```python
from build123d import *

# Parameters (mm, degrees)
SKETCH1_W                      = 3
SKETCH1_H                      = 76
BOSS_EXTRUDE1_DEPTH            = 220
M3_CLEARANCE_HOLE1_D           = 3.4
M3_CLEARANCE_HOLE1_CSINK_D     = 3.45
M3_CLEARANCE_HOLE1_CSINK_ANGLE = 90
SKETCH4_W                      = 220
SKETCH4_H                      = 15
CUT_EXTRUDE1_DEPTH             = 233.776717049
SKETCH5_R                      = 1.75
CUT_EXTRUDE2_DEPTH             = 233.776717049
BOSS_EXTRUDE2_START            = -3
SKETCH6_R                      = 1.725
SKETCH6_R_2                    = 1.7
BOSS_EXTRUDE2_DEPTH            = 3
BOSS_EXTRUDE3_DEPTH            = 3


with BuildPart() as part:
    # Sketch1 → Boss-Extrude1 (new body)
    with BuildSketch(Plane.XY):
        with Locations((1.5, 38)):
            Rectangle(SKETCH1_W, SKETCH1_H)
    extrude(amount=BOSS_EXTRUDE1_DEPTH)

    # M3 Clearance Hole1 (through all)
    with Locations(Plane.ZY):
        with Locations((50.754682085, 59), (60.754682085, 59), (60.754682085, 69), (50.754682085, 69), (200.754682085, 59), (200.754682085, 69), (210.754682085, 59), (210.754682085, 69)):
            CounterSinkHole(M3_CLEARANCE_HOLE1_D / 2, M3_CLEARANCE_HOLE1_CSINK_D / 2, counter_sink_angle=M3_CLEARANCE_HOLE1_CSINK_ANGLE)

    # Sketch4 → Cut-Extrude1 (cut, through all)
    with BuildSketch(Plane.ZY):
        with Locations((110, 7.5)):
            Rectangle(SKETCH4_W, SKETCH4_H)
    extrude(amount=-CUT_EXTRUDE1_DEPTH, mode=Mode.SUBTRACT)

    # Sketch5 → Cut-Extrude2 (cut, through all)
    with BuildSketch(Plane.ZY):
        with Locations((110.754682085, 69)):
            Circle(SKETCH5_R)
        with Locations((100.754682085, 69)):
            Circle(SKETCH5_R)
        with Locations((100.754682085, 59)):
            Circle(SKETCH5_R)
        with Locations((110.754682085, 59)):
            Circle(SKETCH5_R)
    extrude(amount=-CUT_EXTRUDE2_DEPTH, mode=Mode.SUBTRACT)

    # Sketch6 → Boss-Extrude2 (add)
    with BuildSketch(Plane.ZY.offset(BOSS_EXTRUDE2_START)):
        with Locations((50.754682085, 59)):
            Circle(SKETCH6_R)
        with Locations((60.754682085, 59)):
            Circle(SKETCH6_R_2)
        with Locations((60.754682085, 69)):
            Circle(SKETCH6_R)
        with Locations((50.754682085, 69)):
            Circle(SKETCH6_R)
    extrude(amount=BOSS_EXTRUDE2_DEPTH)

    # Sketch7 → Boss-Extrude3 (add)
    with BuildSketch(Plane.ZY):
        Polygon((220, 76), (284, 76), (259.255982343, 45.736716068), (257.707645299, 47.00267515), (247.896462411, 35.003063059), (249.444799455, 33.737103977), (247.387615946, 31.22105628), (249.710121512, 29.322117657), (238, 15), (220, 15), align=None)
    extrude(amount=-BOSS_EXTRUDE3_DEPTH)


solid = part.part
```
Check sheet for the modelled part. Datum: model origin and axes. Units: mm. Give positions to 0.01 mm unless a question says otherwise; leave off trailing zeros. Write each loop counter-clockwise with the first axis right and the second up, starting at its lowest first coordinate (ties: lowest second). Pieces come first, ordered by that corner, then holes. Notation, with made-up numbers: (4, 21) - (47, 21) arc R7 ccw to (47, 31) - close; hole circle Ø7 at (24.25, 10). An arc over 180 degrees is marked (long way). Answer as a JSON object with one key per item and string values. Group by question number.
1) Sectioned sample at B-B (y = 51.5). Record the cut outline in (x, z), then the cut area to 3 significant figures.
2) Sectioned sample at A-A (x = 2.2). Give the number of separate pieces and of enclosed holes in the cut face, then the cut area to 3 significant figures.
3) Sectioned sample at C-C (z = 264). Record the cut outline in (x, y).
4) Depth check by flat-ended pin: P1, Ø4.5, axis at y = 69, z = 110.75, coming from the -X side. Enter the tip coordinate at first touch or a pass-through.
5) Thickness scan on probe 1 along Y at (x, z) = (1.1, 99.5); probe 2 along Z at (x, y) = (2, 69); probe 3 along Z at (x, y) = (0.8, 46). Record the ranges inside material, lowest first. Write a range as from..to.
Geometry results:
{
 "1": {"outline": "(0, 0) - (3, 0) - (3, 263.97) - (0, 263.97) - close", "area": "792 mm^2"},
 "2": {"separate pieces": "1", "enclosed holes": "8", "area": "15,800 mm^2"},
 "3": {"outline": "(0, 51.54) - (3, 51.54) - (3, 76) - (0, 76) - close"},
 "4": {"P1": "stops at x = 0"},
 "5": {"probe 1": "y = 15..57.78, 60.22..67.78, 70.22..76", "probe 2": "z = 0..99, 102.5..109, 112.5..199.05, 202.45..209.05, 212.45..278.28", "probe 3": "z = 0..256.89, 258.93..259.47"}
}
